For this review, take the finished solid that the model builds, in its own axes (mm). Face numbers are marked on the shaded views. A direction names the side the tool comes from. Round coordinates to 2 decimals unless told otherwise and drop trailing zeros. Write each loop counter-clockwise with the first axis right and the second up, starting at its lowest first coordinate (ties: lowest second). Pieces come first, ordered by that corner, then holes.
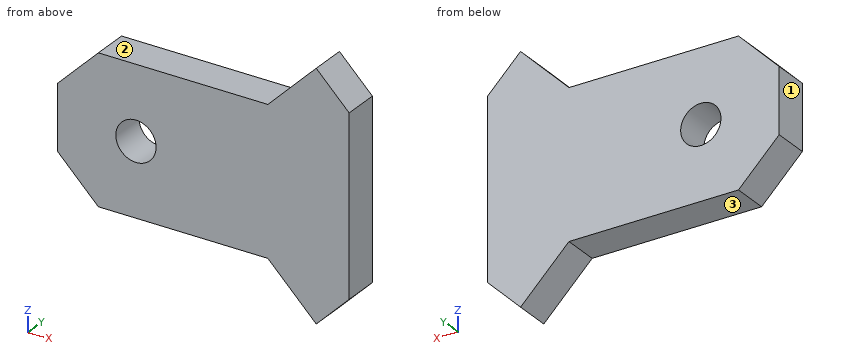
from build123d import *

# Parameters (mm, degrees)
SKETCH1_R           = 2.25
BOSS_EXTRUDE1_DEPTH = 4


with BuildPart() as part:
    # Sketch1 → Boss-Extrude1 (new body)
    with BuildSketch(Plane(origin=(0, 0, 0), x_dir=(1, 0, 0), z_dir=(0, 1, 0))):
        Polygon((0, 3.624368671), (0, -3.624368671), (4.547968979, -8.17233765), (23.47528137, -8.17233765), (23.48528137, -8.18233765), (24.05294372, -8.75), (28.879393916, -13.576450196), (32.556349179, -9.899494934), (32.556349179, 9.899494934), (28.879393916, 13.576450196), (24.05294372, 8.75), (23.48528137, 8.18233765), (23.47528137, 8.17233765), (4.547968979, 8.17233765), align=None)
        with Locations(Location((8.75, 0, 0), (0, 0, 270))):
            Circle(SKETCH1_R, mode=Mode.SUBTRACT)
    extrude(amount=BOSS_EXTRUDE1_DEPTH)


solid = part.part
(1) For line 1 along X through (y, z) = (1.3, 0); line 2 along Z through (x, y) = (12, 3.8); line 3 along X through (y, z) = (0.2, -1), list the stretches that pass through material, from the lowest coordinate up.
Geometry check:
line 1: x = 0 to 6.5, 11 to 32.56
line 2: z = -8.17 to 8.17
line 3: x = 0 to 6.73, 10.77 to 32.56
(2) We need section A-A, the plane x = 8.75. Give the boundary of the cut face in (y, z), and give its area (3 significant figures).
Geometry check:
outline: (0, -8.17) - (4, -8.17) - (4, -2.25) - (0, -2.25) - close; (0, 2.25) - (4, 2.25) - (4, 8.17) - (0, 8.17) - close
area: 47.4 mm2
(3) For pin 1 Ø1.2 at (x, y) = (18, 2.5) entering from +Z; pin 2 Ø1.5 at (y, z) = (3, 9.5) entering from -X, all flat-tipped, find the tip position at first contact; note any pin that passes through.
Geometry check:
pin 1: stops at z = 8.17
pin 2: stops at x = 24.05
(4) We need section C-C, the plane y = 2.95. Give the boundary of the cut face in (x, z), and give its area (3 significant figures).
Geometry check:
outline: (0, -3.62) - (4.55, -8.17) - (23.48, -8.17) - (28.88, -13.58) - (32.56, -9.9) - (32.56, 9.9) - (28.88, 13.58) - (23.48, 8.17) - (4.55, 8.17) - (0, 3.62) - close; hole circle Ø4.5 at (8.75, 0)
area: 551 mm2
(5) We need section D-D, the plane z = 5. Give the boundary of the cut face in (x, y).
Geometry check:
outline: (1.38, 0) - (32.56, 0) - (32.56, 4) - (1.38, 4) - close
(6) We need section B-B, the plane z = 0. Give the boundary of the cut face in (x, y).
Geometry check:
outline: (0, 0) - (6.5, 0) - (6.5, 4) - (0, 4) - close; (11, 0) - (32.56, 0) - (32.56, 4) - (11, 4) - close
(7) For the marked faces 1, 2 and 3, list the 3-axis set-ups (+Z, -Z, +X, -X, +Y, -Y) from which the entire face can be reached by the end or side of a thin tool; tool diameter is ignored.
Geometry check:
face 1: +Z, -Z, -X, +Y, -Y
face 2: +Z, -X, +Y, -Y
face 3: -Z, -X, +Y, -Y
